Check sheet for the modelled part. Datum: model origin and axes. Units: mm. Round coordinates to 2 decimals unless told otherwise and drop trailing zeros. Write each loop counter-clockwise with the first axis right and the second up, starting at its lowest first coordinate (ties: lowest second). Pieces come first, ordered by that corner, then holes.
Item 1: Section check A-A, the plane y = 0. Record the cut outline in (x, z), plus the area to 3 significant figures.
Item 2: Section check D-D, the plane z = 1004. Record the cut outline in (x, y).
Item 3: Depth check by flat-ended pin: pin 1 (1 mm diameter, centred on y = 233, z = 382.5, fed in from -X); pin 2 (2 mm diameter, centred on y = -179.5, z = 1626, fed in from +X); pin 3 (1 mm diameter, centred on x = -180, z = 1751.5, fed in from +Y). Enter the tip coordinate at first touch or a pass-through.
Item 4: Section check B-B, the plane x = 0. Record the cut outline in (y, z).
Item 5: Material ranges on line 1 along X through (y, z) = (-6, 1889) (3 decimals); line 2 along Y through (x, z) = (0, 1159.5); line 3 along Y through (x, z) = (323.5, 376.5), recorded low to high.
Item 6: Release check for a two-part mould opening along X. For faces 1 (the cylindrical face through (216.11, 338.97, 986)), 2 (the cylindrical face through (381.53, 120.15, 986)) record: pulls with the +X half, pulls with the -X half, needs draft (parallel to the pull), parting line crosses it, or undercut.
from build123d import *

# Parameters (mm, degrees)
F0_R      = 402
F0_R_2    = 400
F1_DEPTH  = 2000
F2_R      = 57.5
F3_DEPTH  = 500
F3_FACE_R = 57.5
F4_DEPTH  = 500


with BuildPart() as f1:
    # F0 (on Top) → F1 (new body)
    with BuildSketch(Plane.XY):
        Circle(F0_R)
        Circle(F0_R_2, mode=Mode.SUBTRACT)
    extrude(amount=F1_DEPTH)

    # F2 (on Front) → F3 (join)
    with BuildSketch(Plane.XZ):
        with Locations((0, 110)):
            Circle(F2_R)
    extrude(amount=F3_DEPTH)

    # F3_face (on face) → F4 (cut, through all)
    with BuildSketch(Plane(origin=(0, -500, 110), x_dir=(1, 0, 0), z_dir=(0, -1, 0))):
        Circle(F3_FACE_R)
    extrude(amount=-F4_DEPTH, mode=Mode.SUBTRACT)


solid = f1.part
Values found:
1. outline: (-402, 0) - (-400, 0) - (-400, 2000) - (-402, 2000) - close; (400, 0) - (402, 0) - (402, 2000) - (400, 2000) - close
1. area: 8,000 mm2
2. outline: circle Ø804 at (0, 0); hole circle Ø800 at (0, 0)
3. pin 1: stops at x = -327.94
3. pin 2: stops at x = 360.2
3. pin 3: stops at y = 359.7
4. outline: (-402, 0) - (-400, 0) - (-400, 52.5) - (-402, 52.5) - close; (-402, 167.5) - (-400, 167.5) - (-400, 2000) - (-402, 2000) - close; (400, 0) - (402, 0) - (402, 2000) - (400, 2000) - close
5. line 1: x = -401.955 to -399.955, 399.955 to 401.955
5. line 2: y = -402 to -400, 400 to 402
5. line 3: y = -238.65 to -235.26, 235.26 to 238.65
6. face 1: parting line crosses it
6. face 2: undercut
